Build history of the part. All positions in model axes, mm. Round coordinates to 2 decimals unless told otherwise and drop trailing zeros. Loops run counter-clockwise (first coordinate to the right, second up) from the corner with the lowest first, then second, coordinate; pieces in that order, holes last.
from build123d import *

# Parameters (mm, degrees)
ESQUISSE1_R        = 1.6
BOSS_EXTRU_1_DEPTH = 3


with BuildPart() as part:
    # Esquisse1 → Boss.-Extru.1 (new body)
    with BuildSketch(Plane.XY):
        Polygon((-76.753762562, 51.085106383), (-96.582189687, 51.085106383), (-102.753762562, 44.913533508), (-102.753762562, 35.79522772), (-102.753762562, -22.743320742), (-96.582189687, -28.914893617), (63.932030858, -28.914893617), (73.770824067, -26.278596922), (178.322766002, 34.084494899), (237.005572372, 49.808505475), (241.369533403, 57.367107702), (230.025901746, 99.702117388), (225.368652661, 117.083207596), (223.893223799, 122.719498558), (216.359063387, 127.098384499), (210.670220477, 125.574063635), (147.443918593, 108.632627105), (51.862743071, 53.448809688), (43.041282242, 51.085106383), (-75.988646329, 51.085106383), align=None)
        with Locations((-95.753762562, 44.085106383)):
            Circle(ESQUISSE1_R, mode=Mode.SUBTRACT)
        with Locations((-66.988646329, 44.085106383)):
            Circle(ESQUISSE1_R, mode=Mode.SUBTRACT)
        with Locations((-95.753762562, -21.914893617)):
            Circle(ESQUISSE1_R, mode=Mode.SUBTRACT)
        with Locations((49.263745973, 45.505477252)):
            Circle(ESQUISSE1_R, mode=Mode.SUBTRACT)
        with Locations((67.039694146, -20.835264486)):
            Circle(ESQUISSE1_R, mode=Mode.SUBTRACT)
        with Locations((217.363403759, 120.120565138)):
            Circle(ESQUISSE1_R, mode=Mode.SUBTRACT)
        with Locations((150.12930694, 102.149526137)):
            Circle(ESQUISSE1_R, mode=Mode.SUBTRACT)
        with Locations((175.637377655, 40.567595866)):
            Circle(ESQUISSE1_R, mode=Mode.SUBTRACT)
        with Locations((234.393639901, 56.355573542)):
            Circle(ESQUISSE1_R, mode=Mode.SUBTRACT)
    extrude(amount=BOSS_EXTRU_1_DEPTH)


solid = part.part
(1) Slice it at B-B on z = 0.75. Count the separate pieces of the cut face and the enclosed holes in it, plus the area to 3 significant figures.
Responses:
separate pieces: 1
enclosed holes: 9
area: 28,200 mm2
(2) Slice it at A-A on x = -54.5. List the corners of the cut face in (y, z).
Responses:
outline: (-28.91, 0) - (51.09, 0) - (51.09, 3) - (-28.91, 3) - close
(3) Probe line 1 (Y direction, x = -37.5, z = 1.25); line 2 (X direction, y = -8, z = 1.3); line 3 (X direction, y = 2.5, z = 0.8). List the from-to ranges inside material, lowest first.
Responses:
line 1: y = -28.91 to 51.09
line 2: x = -102.75 to 105.43
line 3: x = -102.75 to 123.62
(4) Pin check, flat tips, straight feed: P1, Ø1, axis at y = 61.5, z = 1, coming from the +X side; P2, Ø1, axis at x = 83.5, z = 2.5, coming from the +Y side. Stop position of each tip, or through.
Responses:
P1: stops at x = 240.4
P2: stops at y = 72
(5) Slice it at C-C on y = -14.5. List the corners of the cut face in (x, z).
Responses:
outline: (-102.75, 0) - (94.17, 0) - (94.17, 3) - (-102.75, 3) - close
